Design review of the part built by this model. Coordinates are the model's own, in mm. Face numbers are marked on the shaded views. A direction names the side the tool comes from. Round coordinates to 2 decimals unless told otherwise and drop trailing zeros. Order: outer loops, then holes, each group sorted by start corner. A loop starts at its lowest first (then second) coordinate and runs counter-clockwise, first axis right, second up. Notation, with made-up numbers: (63.25, -39.75) - (68.25, -39.75) arc R24 cw to (68.25, -1.75) - close; hole circle Ø2 at (38, 85.5). An arc over 180 degrees is marked (long way). Use CSV: the item, a comma, the result in double quotes.
from build123d import *

# Parameters (mm, degrees)
CUT_EXTRUDE1_DEPTH      = 7
CUT_EXTRUDE1_DEPTH_BACK = 7


with BuildPart() as part:
    # Sketch1 → Revolve1 (revolve)
    with BuildSketch(Plane(origin=(0, 0, 0), x_dir=(0, 0, -1), z_dir=(1, 0, 0))):
        with BuildLine():
            Line((0, 0), (6, 0))
            Line((6, 0), (6, -1))
            Line((6, -1), (5, -1))
            Line((5, -1), (4.5, -1.5))
            Line((4.5, -1.5), (5, -2))
            Line((5, -2), (6, -2))
            Line((6, -2), (6, -9))
            ThreePointArc((6, -9), (5.707106781, -9.707106781), (5, -10))
            Line((5, -10), (3, -10))
            Line((3, -10), (2.5, -10.5))
            Line((2.5, -10.5), (2.5, -15.7))
            Line((2.5, -15.7), (2.895480226, -15.7))
            Line((2.895480226, -15.7), (2.5, -17.7))
            Line((2.5, -17.7), (1.5, -17.7))
            Line((1.5, -17.7), (1.5, -10))
            Line((1.5, -10), (0, -10))
            Line((0, -10), (0, 0))
        make_face()
    revolve(axis=Axis((0, -17.7, 0), (0, 1, 0)))

    # Sketch2 → Cut-Extrude1 (cut, two sides)
    with BuildSketch(Plane(origin=(0, -10, 0), x_dir=(-1, 0, 0), z_dir=(0, -1, 0))) as cut_extrude1_sk:
        with BuildLine():
            Line((-1, -14.966629547), (-1, -9.949874371))
            ThreePointArc((-1, -9.949874371), (-2.397127157, -9.708438669), (-3.746065934, -9.271838546))
            Line((-3.746065934, -9.271838546), (-2.13237153, -5.277804741))
            ThreePointArc((-2.13237153, -5.277804741), (-2.474118614, -4.285299143), (-3.504527217, -4.485590286))
            Line((-3.504527217, -4.485590286), (-6.156614753, -7.880107536))
            ThreePointArc((-6.156614753, -7.880107536), (-8.660254038, -5), (-9.902680687, -1.39173101))
            Line((-9.902680687, -1.39173101), (-5.636898747, -0.792214455))
            ThreePointArc((-5.636898747, -0.792214455), (-4.948237227, 0), (-5.636898747, 0.792214455))
            Line((-5.636898747, 0.792214455), (-9.902680687, 1.39173101))
            ThreePointArc((-9.902680687, 1.39173101), (-8.660254038, 5), (-6.156614753, 7.880107536))
            Line((-6.156614753, 7.880107536), (-3.504527217, 4.485590286))
            ThreePointArc((-3.504527217, 4.485590286), (-2.474118614, 4.285299143), (-2.13237153, 5.277804741))
            Line((-2.13237153, 5.277804741), (-3.746065934, 9.271838546))
            ThreePointArc((-3.746065934, 9.271838546), (0, 10), (3.746065934, 9.271838546))
            Line((3.746065934, 9.271838546), (2.13237153, 5.277804741))
            ThreePointArc((2.13237153, 5.277804741), (2.474118614, 4.285299143), (3.504527217, 4.485590286))
            Line((3.504527217, 4.485590286), (6.156614753, 7.880107536))
            ThreePointArc((6.156614753, 7.880107536), (8.660254038, 5), (9.902680687, 1.39173101))
            Line((9.902680687, 1.39173101), (5.636898747, 0.792214455))
            ThreePointArc((5.636898747, 0.792214455), (4.948237227, 0), (5.636898747, -0.792214455))
            Line((5.636898747, -0.792214455), (9.902680687, -1.39173101))
            ThreePointArc((9.902680687, -1.39173101), (8.660254038, -5), (6.156614753, -7.880107536))
            Line((6.156614753, -7.880107536), (3.504527217, -4.485590286))
            ThreePointArc((3.504527217, -4.485590286), (2.474118614, -4.285299143), (2.13237153, -5.277804741))
            Line((2.13237153, -5.277804741), (3.746065934, -9.271838546))
            ThreePointArc((3.746065934, -9.271838546), (1.908089954, -9.816271834), (0, -10))
            Line((0, -10), (0, -15))
            ThreePointArc((0, -15), (0.500278319, 14.991655066), (-1, -14.966629547))
        make_face()
    extrude(amount=CUT_EXTRUDE1_DEPTH, mode=Mode.SUBTRACT)
    extrude(cut_extrude1_sk.sketch, amount=-CUT_EXTRUDE1_DEPTH_BACK, mode=Mode.SUBTRACT)


solid = part.part
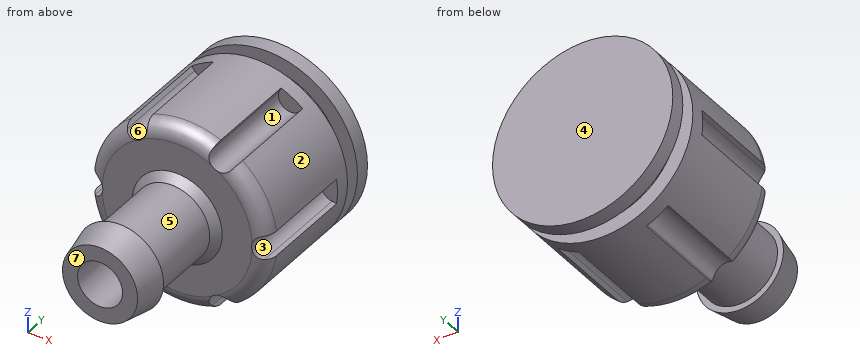
1) For the marked faces 5, 6 and 7, list the 3-axis set-ups (+Z, -Z, +X, -X, +Y, -Y) from which the entire face can be reached by the end or side of a thin tool; tool diameter is ignored.
Data:
face 5,"none"
face 6,"-Y"
face 7,"+Z, -Z, +X, -X, -Y"
2) The part is to be moulded in two halves that separate along X. For the marked faces 1, 2, 3 and 4, say which applies: +X half, -X half, draft (parallel to the pull), parting line (faces both ways), or undercut.
Data:
face 1,"undercut"
face 2,"parting line"
face 3,"+X half"
face 4,"draft"
3) Insertion check: pin 1 Ø4 at (y, z) = (-12.5, 2.5) entering from +X; pin 2 Ø0.7 at (x, z) = (-3, -4.5) entering from -Y; pin 3 Ø0.8 at (x, z) = (5.5, 0) entering from -Y. Each pin has a flat end and moves straight along its axis. Give the tip position at first contact, or say it passes through.
Data:
pin 1,"stops at x = 2.45"
pin 2,"stops at y = -10"
pin 3,"stops at y = -3"
4) To check wall thickness, follow L1, parallel to X at y = -13.5, z = 0; L2, parallel to Y at x = -0.5, z = -5. State the ranges of each line that lie inside material, in increasing order. Write a range as from..to.
Data:
L1,"x = -2.5..-1.5, 1.5..2.5"
L2,"y = -10..-2, -1..0"
5) We need section A-A (y = -11). Give the boundary of the cut face in (x, z).
Data:
outline,"circle Ø5 at (0, 0); hole circle Ø3 at (0, 0)"
6) We need section D-D (y = -6). Give the boundary of the cut face in (x, z).
Data:
outline,"(-5.94, -0.84) arc R6 ccw to (-3.69, -4.73) - (-3.5, -4.49) arc R0.8 cw to (-2.13, -5.28) - (-2.25, -5.56) arc R6 ccw to (2.25, -5.56) - (2.13, -5.28) arc R0.8 cw to (3.5, -4.49) - (3.69, -4.73) arc R6 ccw to (5.94, -0.84) - (5.64, -0.79) arc R0.8 cw to (5.64, 0.79) - (5.94, 0.84) arc R6 ccw to (3.69, 4.73) - (3.5, 4.49) arc R0.8 cw to (2.13, 5.28) - (2.25, 5.56) arc R6 ccw to (-2.25, 5.56) - (-2.13, 5.28) arc R0.8 cw to (-3.5, 4.49) - (-3.69, 4.73) arc R6 ccw to (-5.94, 0.84) - (-5.64, 0.79) arc R0.8 cw to (-5.64, -0.79) - close"
